```python
from build123d import *

# Parameters (mm, degrees)
SKETCH2_W           = 40
SKETCH2_H           = 100
SKETCH2_R           = 5.5
SKETCH2_R_2         = 10.5
BOSS_EXTRUDE1_DEPTH = 100
SKETCH3_R           = 16
CUT_EXTRUDE1_DEPTH  = 4
SKETCH4_R           = 8.05
CUT_EXTRUDE2_DEPTH  = 16
SKETCH5_R           = 1.2
CUT_EXTRUDE3_DEPTH  = 15
CUT_EXTRUDE4_START  = -4
SKETCH6_R           = 16
CUT_EXTRUDE4_DEPTH  = 4
CUT_EXTRUDE5_START  = -16
SKETCH7_R           = 8.05
CUT_EXTRUDE5_DEPTH  = 16
CUT_EXTRUDE6_START  = -15
SKETCH8_R           = 1.2
CUT_EXTRUDE6_DEPTH  = 15


with BuildPart() as part:
    # Sketch2 → Boss-Extrude1 (new body)
    with BuildSketch(Plane.XY):
        with Locations((20, -50)):
            Rectangle(SKETCH2_W, SKETCH2_H)
        with Locations((20, -50)):
            Circle(SKETCH2_R, mode=Mode.SUBTRACT)
        with Locations((20, -20)):
            Circle(SKETCH2_R_2, mode=Mode.SUBTRACT)
        with Locations((20, -80)):
            Circle(SKETCH2_R_2, mode=Mode.SUBTRACT)
    extrude(amount=BOSS_EXTRUDE1_DEPTH)

    # Sketch3 → Cut-Extrude1 (cut)
    with BuildSketch(Plane.XY.offset(100)):
        with Locations((20, -50)):
            Circle(SKETCH3_R)
    extrude(amount=-CUT_EXTRUDE1_DEPTH, mode=Mode.SUBTRACT)

    # Sketch4 → Cut-Extrude2 (cut)
    with BuildSketch(Plane.XY.offset(96)):
        with Locations((20, -50)):
            Circle(SKETCH4_R)
    extrude(amount=-CUT_EXTRUDE2_DEPTH, mode=Mode.SUBTRACT)

    # Sketch5 → Cut-Extrude3 (cut)
    with BuildSketch(Plane.XY.offset(96)):
        with Locations((20, -38)):
            Circle(SKETCH5_R)
        with Locations((8, -50)):
            Circle(SKETCH5_R)
        with Locations((32, -50)):
            Circle(SKETCH5_R)
        with Locations((20, -62)):
            Circle(SKETCH5_R)
    extrude(amount=-CUT_EXTRUDE3_DEPTH, mode=Mode.SUBTRACT)

    # Sketch6 → Cut-Extrude4 (cut)
    with BuildSketch(Plane(origin=(0, 0, 0), x_dir=(-1, 0, 0), z_dir=(0, 0, -1)).offset(CUT_EXTRUDE4_START)):
        with Locations(Location((-20, -50, 0), (0, 0, 180))):
            Circle(SKETCH6_R)
    extrude(amount=CUT_EXTRUDE4_DEPTH, mode=Mode.SUBTRACT)

    # Sketch7 → Cut-Extrude5 (cut)
    with BuildSketch(Plane(origin=(0, 0, 4), x_dir=(-1, 0, 0), z_dir=(0, 0, -1)).offset(CUT_EXTRUDE5_START)):
        with Locations(Location((-20, -50, 0), (0, 0, 180))):
            Circle(SKETCH7_R)
    extrude(amount=CUT_EXTRUDE5_DEPTH, mode=Mode.SUBTRACT)

    # Sketch8 → Cut-Extrude6 (cut)
    with BuildSketch(Plane(origin=(0, 0, 4), x_dir=(-1, 0, 0), z_dir=(0, 0, -1)).offset(CUT_EXTRUDE6_START)):
        with Locations(Location((-20, -62, 0), (0, 0, 180))):
            Circle(SKETCH8_R)
        with Locations(Location((-32, -50, 0), (0, 0, 180))):
            Circle(SKETCH8_R)
        with Locations(Location((-8, -50, 0), (0, 0, 180))):
            Circle(SKETCH8_R)
        with Locations(Location((-20, -38, 0), (0, 0, 180))):
            Circle(SKETCH8_R)
    extrude(amount=CUT_EXTRUDE6_DEPTH, mode=Mode.SUBTRACT)


solid = part.part
```
Verification items for the finished model (mm, model axes). A direction names the side the tool comes from. Give positions to 0.01 mm unless a question says otherwise; leave off trailing zeros. Write each loop counter-clockwise with the first axis right and the second up, starting at its lowest first coordinate (ties: lowest second). Pieces come first, ordered by that corner, then holes. Notation, with made-up numbers: (6, 72.5) - (28, 72.5) arc R22 ccw to (28, 102.5) - close; hole circle Ø3 at (9, 55). An arc over 180 degrees is marked (long way). Put each result on its own line as item: value.
Q1. Section check D-D on x = 20. Count the separate pieces of the cut face and the enclosed holes in it, and give its area (3 significant figures).
Result:
separate pieces: 4
enclosed holes: 0
area: 4,220 mm2
Q2. Section check C-C on z = 60. Record the cut outline in (x, y), and give its area (3 significant figures).
Result:
outline: (0, -100) - (40, -100) - (40, 0) - (0, 0) - close; hole circle Ø21 at (20, -80); hole circle Ø21 at (20, -20); hole circle Ø11 at (20, -50)
area: 3,210 mm2
Q3. Mould release check, pull along Y, two halves, no side actions. Record for faces 4 (the face through (6, -60, 100)), 5 (the face through (7.303, -59.736, 98.028)), 6 (the face through (23, -55, 80)): released by +Y, released by -Y, zero draft, split by the parting line, or undercut.
Result:
face 4: zero draft
face 5: undercut
face 6: undercut
Q4. Section check B-B on z = 87. Record the cut outline in (x, y).
Result:
outline: (0, -100) - (40, -100) - (40, 0) - (0, 0) - close; hole circle Ø2.4 at (8, -50); hole circle Ø21 at (20, -80); hole circle Ø21 at (20, -20); hole circle Ø16.1 at (20, -50); hole circle Ø2.4 at (20, -62); hole circle Ø2.4 at (20, -38); hole circle Ø2.4 at (32, -50)
Q5. Section check A-A on y = -80. Record the cut outline in (x, z), and give its area (3 significant figures).
Result:
outline: (0, 0) - (9.5, 0) - (9.5, 100) - (0, 100) - close; (30.5, 0) - (40, 0) - (40, 100) - (30.5, 100) - close
area: 1,900 mm2
Q6. Scan lines: probe 1 along Y at (x, z) = (20, 79.5); probe 2 along X at (y, z) = (-50, 12); probe 3 along Y at (x, z) = (20, 7.5). Record each from-to range of solid material in increasing order. Write a range as from..to.
Result:
probe 1: -100..-90.5, -69.5..-55.5, -44.5..-30.5, -9.5..0
probe 2: 0..6.8, 9.2..11.95, 28.05..30.8, 33.2..40
probe 3: -100..-90.5, -69.5..-63.2, -60.8..-58.05, -41.95..-39.2, -36.8..-30.5, -9.5..0
Q7. Depth check by flat-ended pin: P1, Ø0.7, axis at x = 19.5, y = -61.5, coming from the -Z side; P2, Ø9.5, axis at x = 20, y = -50, coming from the -Z side; P3, Ø14.5, axis at x = 20, y = -50, coming from the +Z side; P4, Ø17.5, axis at x = 23, y = -53.5, coming from the -Z side. Enter the tip coordinate at first touch or a pass-through.
Result:
P1: z = 19
P2: through
P3: z = 80
P4: z = 4
Q8. Set-up check for faces 1 (the face through (14.067, -44.559, 88.112)), 2 (the face through (23, -45, 20)), 3 (the face through (19.284, -44.547, 49.58)): record each of +Z, -Z, +X, -X, +Y, -Y from which the full face is reachable in a straight line by a thin tool's end or side.
Result:
face 1: +Z
face 2: -Z
face 3: +Z, -Z
